Check sheet for the drawn part. Datum: minimum x, y, z corner. Units: mm. A direction names the side the tool comes from. Give positions to 0.01 mm unless a question says otherwise; leave off trailing zeros. Order: outer loops, then holes, each group sorted by start corner. A loop starts at its lowest first (then second) coordinate and runs counter-clockwise, first axis right, second up.
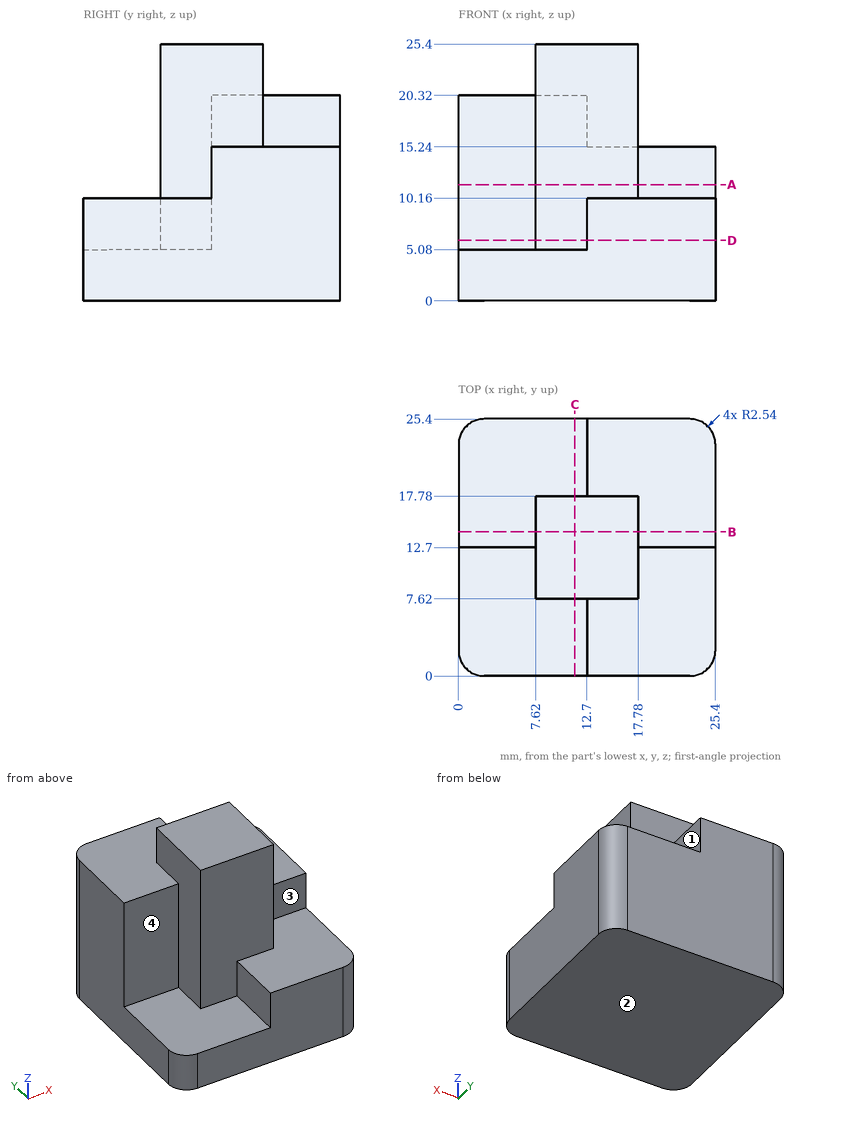
Item 1: Sectioned sample at C-C (x = 11.5). Enter the section's corners in (y, z).
Reported:
outline: (0, 0) - (25.4, 0) - (25.4, 20.32) - (17.78, 20.32) - (17.78, 25.4) - (7.62, 25.4) - (7.62, 5.08) - (0, 5.08) - close
Item 2: Scan lines: L1, parallel to Z at x = 3.75, y = 8.5; L2, parallel to Y at x = 7.25, z = 14.5; L3, parallel to Z at x = 16.5, y = 5.5. Record each from-to range of solid material in increasing order.
Reported:
L1: z = 0 to 5.08
L2: y = 12.7 to 25.4
L3: z = 0 to 10.16
Item 3: Sectioned sample at D-D (z = 6). Enter the section's corners in (x, y), and give its area (3 significant figures).
Reported:
outline: (0, 12.7) - (7.62, 12.7) - (7.62, 7.62) - (12.7, 7.62) - (12.7, 0) - (22.86, 0) arc R2.54 ccw to (25.4, 2.54) - (25.4, 22.86) arc R2.54 ccw to (22.86, 25.4) - (2.54, 25.4) arc R2.54 ccw to (0, 22.86) - close
area: 506 mm2
Item 4: Sectioned sample at B-B (y = 14.25). Enter the section's corners in (x, z).
Reported:
outline: (0, 0) - (25.4, 0) - (25.4, 15.24) - (17.78, 15.24) - (17.78, 25.4) - (7.62, 25.4) - (7.62, 20.32) - (0, 20.32) - close
Item 5: Gauge pin test, flat ends, axial feed: pin 1 (6.5 mm diameter, centred on x = 20, y = 5.5, fed in from +Z); pin 2 (1 mm diameter, centred on x = 5, z = 9, fed in from -Y); pin 3 (2.5 mm diameter, centred on y = 20.5, z = 17, fed in from +X); pin 4 (3 mm diameter, centred on y = 11, z = 20.5, fed in from +X). Record the tip position at first contact, or that the pin passes through.
Reported:
pin 1: stops at z = 25.4
pin 2: stops at y = 12.7
pin 3: stops at x = 12.7
pin 4: stops at x = 17.78
Item 6: Sectioned sample at A-A (z = 11.5). Enter the section's corners in (x, y).
Reported:
outline: (0, 12.7) - (7.62, 12.7) - (7.62, 7.62) - (17.78, 7.62) - (17.78, 12.7) - (25.4, 12.7) - (25.4, 22.86) arc R2.54 ccw to (22.86, 25.4) - (2.54, 25.4) arc R2.54 ccw to (0, 22.86) - close
Item 7: Set-up check for the marked faces 1, 2, 3 and 4: record each of +Z, -Z, +X, -X, +Y, -Y from which the full face is reachable in a straight line by a thin tool's end or side.
Reported:
face 1: +Z, +X, +Y
face 2: -Z, +X, -X, +Y, -Y
face 3: +Z, +X, -Y
face 4: +Z, -X, -Y
